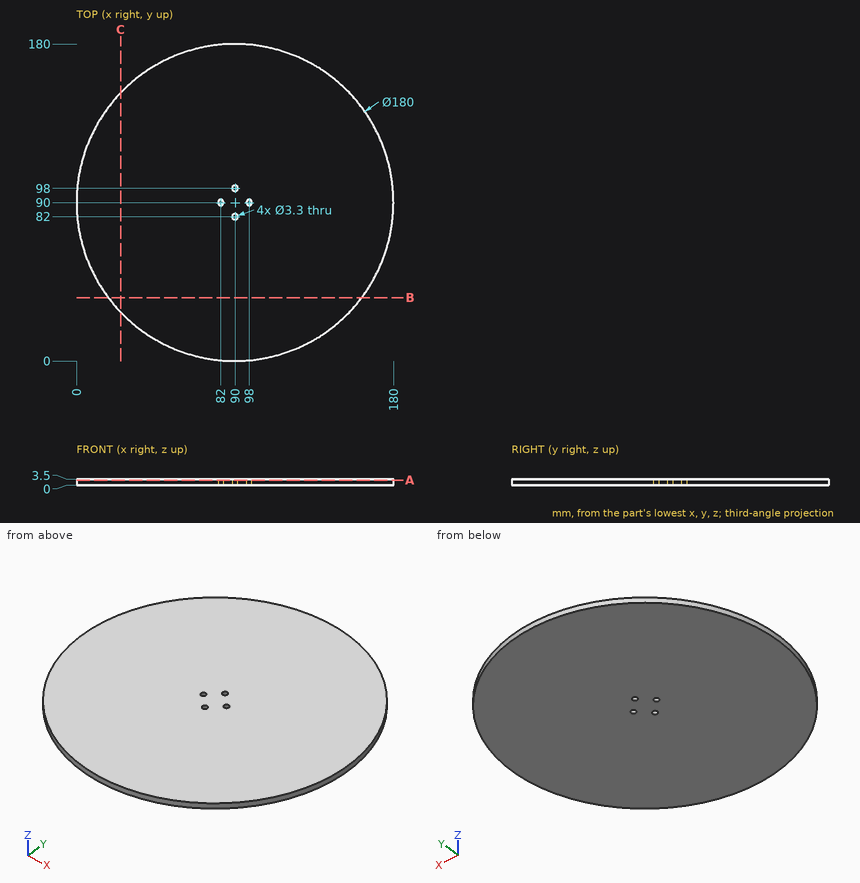
Source: three-view drawing plus pictorial views. Frame: mm from the lowest corner of the part. Round coordinates to 2 decimals unless told otherwise and drop trailing zeros. Loops run counter-clockwise (first coordinate to the right, second up) from the corner with the lowest first, then second, coordinate; pieces in that order, holes last. Notation, with made-up numbers: (26.5, -37) - (48.5, -37) arc R17 ccw to (48.5, -19) - close; hole circle Ø9 at (21.25, 82.25). An arc over 180 degrees is marked (long way). Write item = value, one per line. Start each with the question number.
Item 1: Material intervals for line 1 (Y direction, x = 90, z = 2.5); line 2 (X direction, y = 82, z = 1.8), sorted ascending.
Item 2: Section query B-B on y = 36. Output: boundary loops of the cut face in (x, z).
Item 3: Section query C-C on x = 25. Output: boundary loops of the cut face in (y, z), plus the area to 3 significant figures.
Item 4: First-contact query: pin 1 Ø1.5 at (x, z) = (18.5, 2.5) entering from +Y; pin 2 Ø2 at (x, z) = (86, 1) entering from -Y. Flat tips, straight axial feed; report the tip coordinate or a pass-through.
Item 5: Section query A-A on z = 2.8. Output: boundary loops of the cut face in (x, y).
Results list:
q1.line_1 = 0 to 80.35, 83.65 to 96.35, 99.65 to 180
q1.line_2 = 0.36 to 88.35, 91.65 to 179.64
q2.outline = (18, 0) - (162, 0) - (162, 3.5) - (18, 3.5) - close
q3.outline = (27.75, 0) - (152.25, 0) - (152.25, 3.5) - (27.75, 3.5) - close
q3.area = 436 mm²
q4.pin_1 = 145.63
q4.pin_2 = 0.05
q5.outline = circle Ø180 at (90, 90); hole circle Ø3.3 at (82, 90); hole circle Ø3.3 at (90, 82); hole circle Ø3.3 at (90, 98); hole circle Ø3.3 at (98, 90)
